The listing builds one solid part. Answer for the finished solid, in the listing's coordinates (mm). Face numbers are marked on the shaded views. Coordinates: 2 decimals unless noted, no trailing zeros. Order: outer loops, then holes, each group sorted by start corner. A loop starts at its lowest first (then second) coordinate and runs counter-clockwise, first axis right, second up. Notation, with made-up numbers: (31.5, -15.5) -> (38.5, -15.5) arc R16 cw to (38.5, 7.5) -> close; hole circle Ø7 at (19, -29). An arc over 180 degrees is marked (long way). Return JSON: item names as keys, results as strings.
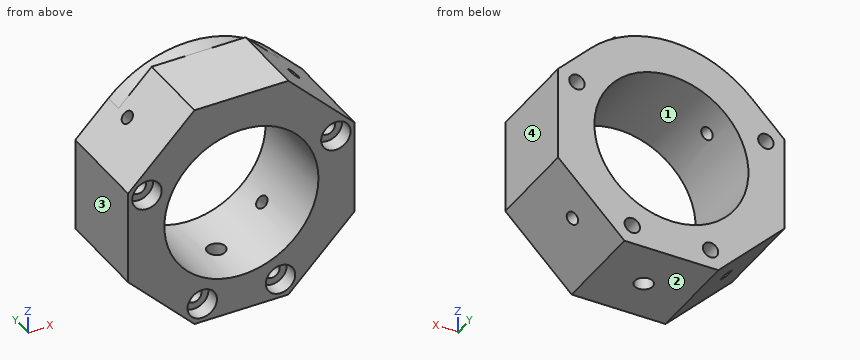
from build123d import *

# Parameters (mm, degrees)
SKETCH1_R                                           = 17
BOSS_EXTRUDE1_DEPTH                                 = 21
CBORE_FOR_M3_HEX_SOCKET_HEAD_CAP_SCREW1_D           = 3.4
CBORE_FOR_M3_HEX_SOCKET_HEAD_CAP_SCREW1_DEPTH       = 21
CBORE_FOR_M3_HEX_SOCKET_HEAD_CAP_SCREW1_CBORE_D     = 6.5
CBORE_FOR_M3_HEX_SOCKET_HEAD_CAP_SCREW1_CBORE_DEPTH = 3.4
M3X0_2_TAPPED_HOLE1_D                               = 2.8
M3X0_2_TAPPED_HOLE2_D                               = 2.8
CUT_EXTRUDE3_REACH                                  = 52
SKETCH12_R                                          = 2
CUT_EXTRUDE4_DEPTH                                  = 4


with BuildPart() as part:
    # Sketch1 → Boss-Extrude1 (new body)
    with BuildSketch(Plane(origin=(0, 0, 0), x_dir=(1, 0, 0), z_dir=(0, 1, 0))):
        Polygon((25, -10.355339059), (25, 10.355339059), (10.355339059, 25), (-10.355339059, 25), (-25, 10.355339059), (-25, -10.355339059), (-10.355339059, -25), (10.355339059, -25), align=None)
        Circle(SKETCH1_R, mode=Mode.SUBTRACT)
    extrude(amount=BOSS_EXTRUDE1_DEPTH)

    # CBORE for M3 Hex Socket Head Cap Screw1
    with Locations(Plane(origin=(0, 0, 0), x_dir=(-1, 0, 0), z_dir=(0, -1, 0))):
        with Locations((20.842542104, -8.633263614), (-20.842542104, -8.633263614), (8.633263614, 20.842542104), (-8.633263614, 20.842542104)):
            CounterBoreHole(CBORE_FOR_M3_HEX_SOCKET_HEAD_CAP_SCREW1_D / 2, CBORE_FOR_M3_HEX_SOCKET_HEAD_CAP_SCREW1_CBORE_D / 2, CBORE_FOR_M3_HEX_SOCKET_HEAD_CAP_SCREW1_CBORE_DEPTH, depth=CBORE_FOR_M3_HEX_SOCKET_HEAD_CAP_SCREW1_DEPTH)

    # M3x0.2 Tapped Hole1 (through all)
    with Locations(Plane(origin=(17.67766953, 0, 17.67766953), x_dir=(0.707106781, 0, -0.707106781), z_dir=(0.707106781, 0, 0.707106781))):
        with Locations((0, 11)):
            Hole(M3X0_2_TAPPED_HOLE1_D / 2)

    # M3x0.2 Tapped Hole2 (through all)
    with Locations(Plane(origin=(-17.67766953, 0, 17.67766953), x_dir=(0.707106781, 0, 0.707106781), z_dir=(-0.707106781, 0, 0.707106781))):
        with Locations((0, 13.5)):
            Hole(M3X0_2_TAPPED_HOLE2_D / 2)

    # Sketch12 → Cut-Extrude3 (cut, up to next)
    with BuildSketch(Plane(origin=(0, 0, -25), x_dir=(-1, 0, 0), z_dir=(0, 0, -1)), mode=Mode.PRIVATE) as cut_extrude3_sk1:
        with Locations((0, 10)):
            Circle(SKETCH12_R)
    cut_extrude3_tool1 = extrude(cut_extrude3_sk1.sketch, amount=-CUT_EXTRUDE3_REACH, mode=Mode.PRIVATE) & part.part
    add(cut_extrude3_tool1.solids().sort_by_distance((0, 10, -25))[0], mode=Mode.SUBTRACT)

    # Sketch13 → Cut-Extrude4 (cut)
    with BuildSketch(Plane(origin=(0, 21, 0), x_dir=(1, 0, 0), z_dir=(0, 1, 0))):
        with BuildLine():
            Line((17.67766953, -17.67766953), (17.67766953, -26.659644855))
            Line((17.67766953, -26.659644855), (-17.67766953, -26.659644855))
            Line((-17.67766953, -26.659644855), (-17.67766953, -17.67766953))
            ThreePointArc((-17.67766953, -17.67766953), (0, -25), (17.67766953, -17.67766953))
        make_face()
    extrude(amount=-CUT_EXTRUDE4_DEPTH, mode=Mode.SUBTRACT)


solid = part.part
1. Determine the mould class of the marked faces 1, 2, 3 and 4 for opening direction X: pulls with the +X half, pulls with the -X half, needs draft (parallel to the pull), parting line crosses it, or undercut.
Answer block:
{"face 1": "undercut", "face 2": "needs draft", "face 3": "pulls with the -X half", "face 4": "pulls with the +X half"}
2. Consider line 1 (Z direction, x = -9, y = 9); line 2 (X direction, y = 8.25, z = -22); line 3 (X direction, y = 1.5, z = 9.5). Determine where each line is inside the solid, lowest interval first. Write a range as from..to.
Answer block:
{"line 1": "z = -25..-22.5, -19.18..-14.42, 14.42..25", "line 2": "x = -13.36..-9.88, -7.39..-0.97, 0.97..7.39, 9.88..13.36", "line 3": "x = -25..-23.97, -17.71..-14.1, 14.1..17.71, 23.97..25"}
3. The part is cut by section A-A on z = 0. Give the vertices of the cut face in (x, y), and give its area (3 significant figures).
Answer block:
{"outline": "(-25, 0) -> (-17, 0) -> (-17, 21) -> (-25, 21) -> close; (17, 0) -> (25, 0) -> (25, 21) -> (17, 21) -> close", "area": "336 mm2"}
4. Each of these flat-tipped pins is pushed along its axis until it touches: pin 1 Ø2 at (x, z) = (-21, 7.5) entering from -Y; pin 2 Ø1 at (y, z) = (12.5, 17.5) entering from -X; pin 3 Ø3.5 at (x, y) = (0, 10) entering from -Z. Where does it stop, or does it pass through?
Answer block:
{"pin 1": "stops at y = 3.4", "pin 2": "stops at x = -18.35", "pin 3": "stops at z = 16.91"}
5. The part is cut by section B-B on x = -4. Give the vertices of the cut face in (y, z).
Answer block:
{"outline": "(0, -25) -> (21, -25) -> (21, -16.52) -> (0, -16.52) -> close; (0, 16.52) -> (21, 16.52) -> (21, 24.68) -> (17, 24.68) -> (17, 25) -> (0, 25) -> close"}
6. The part is cut by section D-D on z = 21.5. Give the vertices of the cut face in (x, y), and give its area (3 significant figures).
Answer block:
{"outline": "(-13.86, 0) -> (13.86, 0) -> (13.86, 17) -> (12.76, 17) -> (12.76, 21) -> (-12.76, 21) -> (-12.76, 17) -> (-13.86, 17) -> close", "area": "573 mm2"}
7. The part is cut by section C-C on y = 2.25. Give the vertices of the cut face in (x, z), and give its area (3 significant figures).
Answer block:
{"outline": "(-25, -10.36) -> (-10.36, -25) -> (10.36, -25) -> (25, -10.36) -> (25, 10.36) -> (10.36, 25) -> (-10.36, 25) -> (-25, 10.36) -> close; hole circle Ø6.5 at (-20.84, 8.63); hole circle Ø34 at (0, 0); hole circle Ø6.5 at (-8.63, -20.84); hole circle Ø6.5 at (8.63, -20.84); hole circle Ø6.5 at (20.84, 8.63)", "area": "1,030 mm2"}
